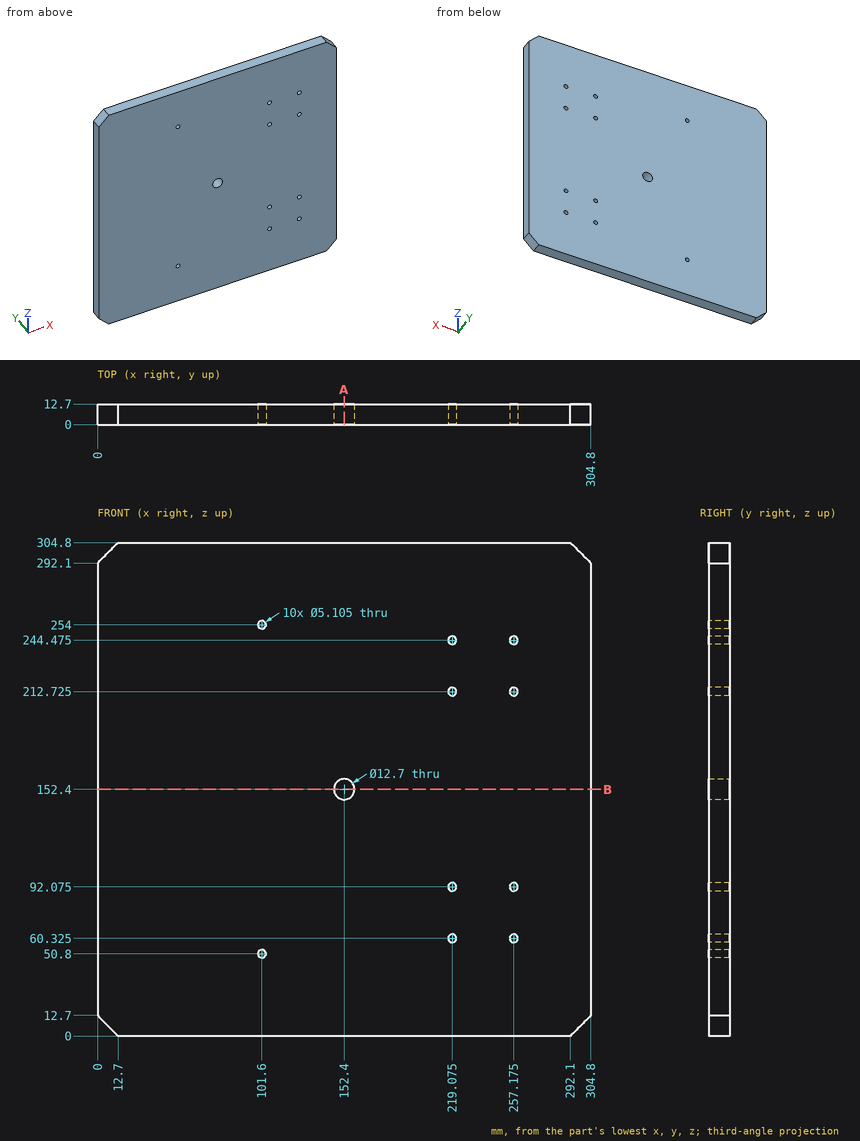
Verification items for this drawing (mm, ordinates from the low corner). Give positions to 0.01 mm unless a question says otherwise; leave off trailing zeros. Loops run counter-clockwise (first coordinate to the right, second up) from the corner with the lowest first, then second, coordinate; pieces in that order, holes last.
1. Cross-section at A-A on x = 152.4. Record the cut outline in (y, z), and give its area (3 significant figures).
Derived:
outline: (0, 0) - (12.7, 0) - (12.7, 146.05) - (0, 146.05) - close; (0, 158.75) - (12.7, 158.75) - (12.7, 304.8) - (0, 304.8) - close
area: 3,710 mm2
2. Material ranges on probe 1 along Z at (x, y) = (101.6, 9.5); probe 2 along X at (y, z) = (7.5, 152.4), recorded low to high.
Derived:
probe 1: z = 0 to 48.25, 53.35 to 251.45, 256.55 to 304.8
probe 2: x = 0 to 146.05, 158.75 to 304.8
3. Go/stop test with flat-tipped pins: P1, Ø3, axis at x = 257.175, z = 244.475, coming from the -Y side; P2, Ø6, axis at x = 257.175, z = 212.725, coming from the -Y side. Record where each tip stops, or that it passes through.
Derived:
P1: passes through
P2: stops at y = 0
4. Cross-section at B-B on z = 152.4. Record the cut outline in (x, y).
Derived:
outline: (0, 0) - (146.05, 0) - (146.05, 12.7) - (0, 12.7) - close; (158.75, 0) - (304.8, 0) - (304.8, 12.7) - (158.75, 12.7) - close
